Geometry check sheet. Reference: the model listing, model coordinates, mm. Face numbers are marked on the shaded views. A direction names the side the tool comes from. Round coordinates to 2 decimals unless told otherwise and drop trailing zeros. Loops run counter-clockwise (first coordinate to the right, second up) from the corner with the lowest first, then second, coordinate; pieces in that order, holes last. Notation, with made-up numbers: M 37,61 L 74,61 A31 ccw 74,100 Z; hole C 42.5,7 d10. An arc over 180 degrees is marked long. Answer in a Markdown table with one row per item. Add a question column.
```python
from build123d import *

# Parameters (mm, degrees)
F1_DEPTH      = 5
F4_DEPTH      = 2
F4_DEPTH_BACK = 7
F6_DEPTH      = 25
F7_SIZE       = 2
F8_SIZE       = 0.99999
F10_DEPTH     = 19
F11_SIZE      = 1


# Not quite as in the source:
# - a fillet or chamfer is up to 0.001 mm smaller than in the source, because OpenCascade refuses the exact size


with BuildPart() as f1:
    # F0 (on Front) → F1 (new body)
    with BuildSketch(Plane.XZ):
        Polygon((0, 28), (0, 0), (10, 0), (10, 31.5), (4, 31.5), (4, 41), (-1, 41), (-1, 28), align=None)
        with BuildLine():
            ThreePointArc((3.4, 6.1), (5, 7.7), (6.6, 6.1))
            Line((6.6, 6.1), (6.6, 2.9))
            ThreePointArc((6.6, 2.9), (5, 1.3), (3.4, 2.9))
            Line((3.4, 2.9), (3.4, 6.1))
        make_face(mode=Mode.SUBTRACT)
    extrude(amount=F1_DEPTH)

    # F3 (on face) → F4 (join, two sides)
    with BuildSketch(Plane(origin=(0, 0, 0), x_dir=(-1, 0, 0), z_dir=(0, 1, 0))) as f4_sk:
        Polygon((1, 28), (1, 41), (-4, 41), (-4, 31.5), (-4, 28), (0, 28), align=None)
    extrude(amount=F4_DEPTH)
    extrude(f4_sk.sketch, amount=-F4_DEPTH_BACK)

    # F5 (on face) → F6 (cut)
    with BuildSketch(Plane(origin=(-1, 0, 0), x_dir=(0, -1, 0), z_dir=(-1, 0, 0))):
        with BuildLine():
            Line((3.6, 34.9), (3.6, 38.1))
            ThreePointArc((3.6, 38.1), (2, 39.7), (0.4, 38.1))
            Line((0.4, 38.1), (0.4, 34.9))
            ThreePointArc((0.4, 34.9), (2, 33.3), (3.6, 34.9))
        make_face()
    extrude(amount=-F6_DEPTH, mode=Mode.SUBTRACT)

    # F7
    f7_edges = [f1.edges().sort_by_distance(p)[0] for p in [
        (1.5, 2, 28),
        (1.5, -7, 28),
    ]]
    chamfer(f7_edges, length=F7_SIZE)

    # F8 (size 1 in the source; OpenCascade refuses exactly that, so slightly less here)
    f8_edges = [f1.edges().sort_by_distance(p)[0] for p in [
        (-1, -2.5, 28),
    ]]
    chamfer(f8_edges, length=F8_SIZE)

    # F9 (on offset) → F10 (cut)
    with BuildSketch(Plane.XY.offset(9)):
        with BuildLine():
            Line((10, 0), (7, 0))
            ThreePointArc((7, 0), (9.1213203436, -0.8786796564), (10, -3))
            Line((10, -3), (10, 0))
        make_face()
        with BuildLine():
            ThreePointArc((0, -3), (0.8786796564, -0.8786796564), (3, 0))
            Line((3, 0), (0, 0))
            Line((0, 0), (0, -3))
        make_face()
    extrude(amount=F10_DEPTH, mode=Mode.SUBTRACT)

    # F11
    f11_edges = [f1.edges().sort_by_distance(p)[0] for p in [
        (6.6, 0, 4.5),
        (-1, -3.6, 36.5),
    ]]
    chamfer(f11_edges, length=F11_SIZE)


solid = f1.part
```
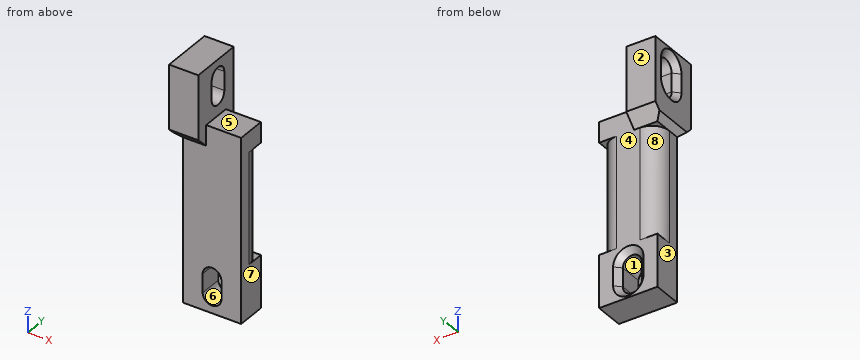
1) Draft check along Z on the marked faces 5, 6, 7 and 8. Enter one of: +Z half, -Z half, draft (parallel to the pull), parting line (faces both ways), or undercut.
2) Set-up check for the marked faces 1, 2, 3 and 4: record each of +Z, -Z, +X, -X, +Y, -Y from which the full face is reachable in a straight line by a thin tool's end or side.
3) Cross-section at A-A, the plane x = 5. Record the boundary of the cut face in (y, z), plus the area to 4 significant figures.
4) Cross-section at D-D, the plane z = 17.5. Record the boundary of the cut face in (x, y).
5) Cross-section at C-C, the plane y = -2.5. Count the separate pieces of the cut face and the enclosed holes in it, plus the area to 3 significant figures.
6) Go/stop test with flat-tipped pins: pin 1 (3 mm diameter, centred on x = 7.5, z = 14.5, fed in from -Y); pin 2 (4.5 mm diameter, centred on y = -4, z = 34, fed in from +X); pin 3 (2.5 mm diameter, centred on x = 6.5, y = -3.5, fed in from +Z). Record where each tip stops, or that it passes through.
7) Cross-section at B-B, the plane z = 35.5. Record the boundary of the cut face in (x, y), plus the area to 3 significant figures.
8) Thickness scan on L1, parallel to Y at x = 3.25, z = 38; L2, parallel to X at y = -3.25, z = 27.5; L3, parallel to Y at x = 6, z = 25. Record the ranges inside material, lowest first. Write a range as [from, to].
Worked answers:
| question | item | result |
|---|---|---|
| 1 | face 5 | +Z half |
| 1 | face 6 | undercut |
| 1 | face 7 | draft |
| 1 | face 8 | undercut |
| 2 | face 1 | +Y, -Y |
| 2 | face 2 | +Z, -Z, +X, -X, +Y |
| 2 | face 3 | -Z, -X, +Y, -Y |
| 2 | face 4 | -Z, +X, +Y |
| 3 | outline | M -5,0 L 0,0 L 0,0.3 L -1,1.3 L -5,1.3 Z; M -5,7.7 L -1,7.7 L 0,8.7 L 0,31.5 L -5,31.5 Z |
| 3 | area | 124.5 mm2 |
| 4 | outline | M 0,-5 L 10,-5 L 10,-3 A3 ccw 7,0 L 3,0 A3 ccw 0,-3 Z |
| 5 | separate pieces | 2 |
| 5 | enclosed holes | 1 |
| 5 | area | 313 mm2 |
| 6 | pin 1 | stops at y = -5 |
| 6 | pin 2 | stops at x = 4 |
| 6 | pin 3 | stops at z = 31.5 |
| 7 | outline | M -1,-7 L 4,-7 L 4,-3.6 L 0,-3.6 L -1,-4.6 Z; M -1,0.6 L 0,-0.4 L 4,-0.4 L 4,2 L -1,2 Z |
| 7 | area | 28.0 mm2 |
| 8 | L1 | y = [-7, -3.6], [-0.4, 2] |
| 8 | L2 | x = [0, 10] |
| 8 | L3 | y = [-5, 0] |
